Read the model definition and answer for the solid it produces. Units are mm, in the model's axes. A direction names the side the tool comes from. Coordinates: 2 decimals unless noted, no trailing zeros. Write each loop counter-clockwise with the first axis right and the second up, starting at its lowest first coordinate (ties: lowest second). Pieces come first, ordered by that corner, then holes.
(1) The part is cut by section C-C, the plane y = 2.5. Determine the outline of the cut face in (x, z), and give its area (3 significant figures).
(2) Straight lines are drawn through the part: line 1 along X through (y, z) = (9, 0); line 2 along Z through (x, y) = (2, 2). For each, find the intervals that lie inside material, in ascending order.
(3) The part is cut by section D-D, the plane y = 12.25. Determine the outline of the cut face in (x, z), and give its area (3 significant figures).
(4) The part is cut by section B-B, the plane x = 0. Determine the outline of the cut face in (y, z), and give its area (3 significant figures).
(5) Which of the six approach directions +Z, -Z, +X, -X, +Y, -Y give full straight-line access (tool end or side, diameter ignored) to faces 4 (the flat face through (-1, 0, -3.5)), 5 (the cylindrical face through (1.08, 7.4, 4.88))?
(6) Given pin 1 (4 mm diameter, centred on y = 2.5, z = -6.5, fed in from +X); pin 2 (4 mm diameter, centred on y = 11, z = -4.5, fed in from -X); pin 3 (4.5 mm diameter, centred on x = -1.5, z = -7.5, fed in from +Y), each flat-ended and moving along its own axis, determine where each tip first touches the part or whether it passes through.
(7) Determine the mould class of faces 1 (the flat face through (0, 5, -7)), 2 (the flat face through (0, 2, -9)), 3 (the cylindrical face through (0.74, 7.4, 3.32)) for opening direction Z: pulls with the +Z half, pulls with the -Z half, needs draft (parallel to the pull), parting line crosses it, or undercut.
(8) The part is cut by section A-A, the plane z = 0. Determine the outline of the cut face in (x, y), and give its area (3 significant figures).
Autodesk Inventor part; units mm, degrees
ref_plane "YZ Plane" through (0, 0, 0) normal (1, 0, 0) x (0, 1, 0)
ref_plane "XZ Plane" through (0, 0, 0) normal (0, 1, 0) x (-1, 0, 0)
ref_plane "XY Plane" through (0, 0, 0) normal (0, 0, 1) x (1, 0, 0)
sketch "Sketch1" plane through (0, 0, 0) normal (0, 1, 0) x (-1, 0, 0)
  circle A0 centre (0, 0) radius 3.4
  circle A1 centre (0, 0) radius 5
  line L0 (3.4, 0) -> (3.4, -9)
  line L1 (3.4, -9) -> (-3.4, -9)
  line L2 (-3.4, -9) -> (-3.4, 0)
  dimension "d0" = 6.8
  dimension "d1" = 10
  dimension "d2" = 9
extrude "Extrusion1" add sketch "Sketch1" along normal blind 5 contours L0 A1 L2 A0 | L0 L1 L2 A1 picked at (2.574, -3.6186)
extrude "Extrusion2" add sketch "Sketch1" along normal blind 15 contours L0 A1 L2 A0 | A0 L2 A1 L0
sketch "Sketch2" plane through (3.4, 0, -9) normal (1, 0, 0) x (0, 0, -1)
  line L0 (0, 5) -> (0, 2.5)
  line L1 (0, 0) -> (0, 5)
  line L2 (0, 2.5) -> (-2, 2.5)
  circle A0 centre (-2, 2.5) radius 1.55
  circle A1 centre (-2, 2.5) radius 4
  point P0 (-9, 0)
  dimension "d7" = 2.5
  dimension "d8" = 2
  dimension "d9" = 3.1
  dimension "d10" = 8
extrude "Extrusion3" cut sketch "Sketch2" against normal blind 15 contours A0
extrude "Extrusion4" cut sketch "Sketch2" along normal blind 15
sketch "Sketch3" plane through (-3.4, 0, -9) normal (-1, 0, 0) x (0, 0, 1)
  line L0 (0, 5) -> (2, 5)
  line L1 (0, 5) -> (5.3339, 5)
  line L2 (2, 5) -> (2, 2.5)
  circle A0 centre (2, 2.5) radius 4
  point P0 (9, 0)
  dimension "d15" = 2
  dimension "d16" = 2.5
  dimension "d17" = 8
extrude "Extrusion5" cut sketch "Sketch3" along normal blind 15
properties part number "push_clip(2)"
Computed:
1. outline: (-4, -3) - (-3.4, -3) - (-3.4, -5.45) - (3.4, -5.45) - (3.4, -3) - (4, -3) arc R5 ccw (long way) to start; (-3.4, -9) - (3.4, -9) - (3.4, -8.55) - (-3.4, -8.55) - close; hole circle Ø6.8 at (0, 0)
1. area: 50.8 mm2
2. line 1: x = -5 to -3.4, 3.4 to 5
2. line 2: z = -9 to -8.47, -5.53 to -2.75, 2.75 to 4.58
3. outline: circle Ø10 at (0, 0); hole circle Ø6.8 at (0, 0)
3. area: 42.2 mm2
4. outline: (0, -9) - (5, -9) - (5, -5) - (15, -5) - (15, -3.4) - (0, -3.4) - close; (0, 3.4) - (15, 3.4) - (15, 5) - (0, 5) - close; hole circle Ø3.1 at (2.5, -7)
4. area: 60.5 mm2
5. face 4: +Z, -Z, +X, -X, -Y
5. face 5: +Y
6. pin 1: stops at x = 3.4
6. pin 2: stops at x = -4.33
6. pin 3: stops at y = 5
7. face 1: needs draft
7. face 2: pulls with the -Z half
7. face 3: undercut
8. outline: (-5, 0) - (-3.4, 0) - (-3.4, 15) - (-5, 15) - close; (3.4, 0) - (5, 0) - (5, 15) - (3.4, 15) - close
8. area: 48.0 mm2
